```python
from build123d import *

# Parameters (mm, degrees)
SKETCH1_W           = 15
SKETCH1_H           = 28
SKETCH1_R           = 4
BOSS_EXTRUDE1_DEPTH = 10
SKETCH2_W           = 15
SKETCH2_H           = 28
BOSS_EXTRUDE2_DEPTH = 20
CUT_EXTRUDE1_DEPTH  = 15
CHAMFER1_SIZE       = 2


with BuildPart() as part:
    # Sketch1 → Boss-Extrude1 (new body)
    with BuildSketch(Plane(origin=(0, 0, 0), x_dir=(1, 0, 0), z_dir=(0, 1, 0))):
        with Locations((-0.01385015, -0.098387905)):
            Rectangle(SKETCH1_W, SKETCH1_H)
        with Locations(Location((0, 8, 0), (0, 0, 270))):
            Circle(SKETCH1_R, mode=Mode.SUBTRACT)
        with Locations(Location((0, -8, 0), (0, 0, 90))):
            Circle(SKETCH1_R, mode=Mode.SUBTRACT)
    extrude(amount=BOSS_EXTRUDE1_DEPTH)

    # Sketch2 → Boss-Extrude2 (add)
    with BuildSketch(Plane(origin=(0, 10, 0), x_dir=(1, 0, 0), z_dir=(0, 1, 0))):
        with Locations((-0.01385015, -0.098387905)):
            Rectangle(SKETCH2_W, SKETCH2_H)
    extrude(amount=BOSS_EXTRUDE2_DEPTH)

    # Sketch3 → Cut-Extrude1 (cut)
    with BuildSketch(Plane(origin=(0, 30, 0), x_dir=(1, 0, 0), z_dir=(0, 1, 0))):
        Polygon((-3.103489636, 9.215029418), (-1.103489636, 11.215029418), (1.103489636, 11.215029418), (3.103489636, 9.215029418), (3.103489636, 6.25292645), (1.103489636, 4.25292645), (-1.103489636, 4.25292645), (-3.103489636, 6.25292645), align=None)
        Polygon((-1.103489636, -4.25292645), (1.103489636, -4.25292645), (3.103489636, -6.25292645), (3.103489636, -9.215029418), (1.103489636, -11.215029418), (-1.103489636, -11.215029418), (-3.103489636, -9.215029418), (-3.103489636, -6.25292645), align=None)
    extrude(amount=-CUT_EXTRUDE1_DEPTH, mode=Mode.SUBTRACT)

    # Chamfer1
    chamfer1_edges = [part.edges().sort_by_distance(p)[0] for p in [
        (7.48614985, 15, 14.098387905),
        (-7.51385015, 15, 14.098387905),
        (-7.51385015, 15, -13.901612095),
        (7.48614985, 15, -13.901612095),
    ]]
    chamfer(chamfer1_edges, length=CHAMFER1_SIZE)


solid = part.part
```
The listing builds one solid part. Answer for the finished solid, in the listing's coordinates (mm). A direction names the side the tool comes from. Round coordinates to 2 decimals unless told otherwise and drop trailing zeros. Loops run counter-clockwise (first coordinate to the right, second up) from the corner with the lowest first, then second, coordinate; pieces in that order, holes last. Notation, with made-up numbers: (-16, 39) - (42, 39) arc R31 cw to (42, 78) - close; hole circle Ø3 at (-35.75, 61). An arc over 180 degrees is marked (long way). Return JSON: item names as keys, results as strings. Group by question number.
1. Each of these flat-tipped pins is pushed along its axis until it touches: P1, Ø1.9, axis at x = 0, z = 8, coming from the +Y side; P2, Ø5, axis at x = -1, z = -9, coming from the +Y side; P3, Ø2.5, axis at x = -0.5, z = 8.5, coming from the -Y side. Where does it stop, or does it pass through?
2. The mould has two halves that part along X. Classify faces 4 (the flat face through (0, 15, -13.902)), 5 (the flat face through (-3.103, 23, -8)), 6 (the flat face through (6.5, 14.79, 13.084)), 7 (the cylindrical face through (2.4, 4.9, 11.2)): pulls with the +X half, pulls with the -X half, needs draft (parallel to the pull), parting line crosses it, or undercut.
3. Consider probe 1 along X at (y, z) = (6.5, 8); probe 2 along Y at (x, z) = (1.75, -5.25); probe 3 along Y at (x, z) = (-3.25, -5.75). Determine where each line is inside the solid, lowest interval first.
4. The part is cut by section B-B on z = -7. Determine the outline of the cut face in (x, y).
5. The part is cut by section A-A on y = 9. Determine the outline of the cut face in (x, z), then the cut area to 3 significant figures.
6. The part is cut by section D-D on y = 13.75. Determine the outline of the cut face in (x, z), then the cut area to 3 significant figures.
7. The part is cut by section C-C on x = 0. Determine the outline of the cut face in (y, z), then the cut area to 3 significant figures.
8. Which of the six approach directions +Z, -Z, +X, -X, +Y, -Y give full straight-line access (tool end or side, diameter ignored) to faces 1 (the flat face through (0, 10, -8)), 2 (the flat face through (0, 23, 11.215)), 3 (the flat face through (0, 0, 0))?
Resolved:
{
 "1": {"P1": "stops at y = 15", "P2": "stops at y = 30", "P3": "stops at y = 10"},
 "2": {"face 4": "needs draft", "face 5": "undercut", "face 6": "pulls with the +X half", "face 7": "undercut"},
 "3": {"probe 1": "x = -7.51 to -4, 4 to 7.49", "probe 2": "y = 10 to 15", "probe 3": "y = 10 to 30"},
 "4": {"outline": "(-7.51, 0) - (-3.87, 0) - (-3.87, 10) - (3.87, 10) - (3.87, 0) - (7.49, 0) - (7.49, 30) - (3.1, 30) - (3.1, 15) - (-3.1, 15) - (-3.1, 30) - (-7.51, 30) - close"},
 "5": {"outline": "(-7.51, -11.9) - (-5.51, -13.9) - (5.49, -13.9) - (7.49, -11.9) - (7.49, 12.1) - (5.49, 14.1) - (-5.51, 14.1) - (-7.51, 12.1) - close; hole circle Ø8 at (0, -8); hole circle Ø8 at (0, 8)", "area": "311 mm²"},
 "6": {"outline": "(-7.51, -11.9) - (-5.51, -13.9) - (5.49, -13.9) - (7.49, -11.9) - (7.49, 12.1) - (5.49, 14.1) - (-5.51, 14.1) - (-7.51, 12.1) - close", "area": "412 mm²"},
 "7": {"outline": "(0, -13.9) - (30, -13.9) - (30, -11.22) - (15, -11.22) - (15, -4.25) - (30, -4.25) - (30, 4.25) - (15, 4.25) - (15, 11.22) - (30, 11.22) - (30, 14.1) - (0, 14.1) - (0, 12) - (10, 12) - (10, 4) - (0, 4) - (0, -4) - (10, -4) - (10, -12) - (0, -12) - close", "area": "471 mm²"},
 "8": {"face 1": "-Y", "face 2": "+Y", "face 3": "+Z, -Z, +X, -X, -Y"}
}
